Source: CAD feature listing. Evaluate the final solid. Frame: model axes, mm. A direction names the side the tool comes from. Round coordinates to 2 decimals unless told otherwise and drop trailing zeros. Loops run counter-clockwise (first coordinate to the right, second up) from the corner with the lowest first, then second, coordinate; pieces in that order, holes last. Notation, with made-up numbers: M -39,-32 L -11,-32 A17 ccw -11,-11 Z; hole C 45.5,-22.5 d1. An arc over 180 degrees is marked long. Answer as a JSON object with one key per item and string values.
from build123d import *

# Parameters (mm, degrees)
F1_DEPTH = 50.8
F3_DEPTH = 2.54
F4_W     = 170.18
F4_H     = 43.18
F5_DEPTH = 82.5510001


with BuildPart() as f1:
    # F0 (on Front) → F1 (new body)
    with BuildSketch(Plane.XZ):
        with BuildLine():
            Line((-89.1799991712, 82.55), (-89.1799991712, 0))
            Line((-89.1799991712, 0), (88.6200008288, 0))
            Line((88.6200008288, 0), (88.6200008288, 82.55))
            Line((88.6200008288, 82.55), (85.1941899427, 82.55))
            ThreePointArc((85.1941899427, 82.55), (0, 6.35), (-85.1941899427, 82.55))
            Line((-85.1941899427, 82.55), (-89.1799991712, 82.55))
        make_face()
    extrude(amount=F1_DEPTH)

    # F2 (on face) → F3 (cut)
    with BuildSketch(Plane.YZ.offset(88.6200008288)):
        Polygon((-37.5634527076, 56.1206514695), (-45.9675195587, 33.2813703549), (-43.8684808629, 33.2813703549), (-35.4644140118, 56.1206514695), align=None)
        Polygon((-37.9258376017, 33.2813703549), (-30.8785599801, 33.2813703549), (-22.4744931291, 56.1206514695), (-29.5217707507, 56.1206514695), align=None)
        Polygon((-34.8114763209, 56.1206514695), (-43.215543172, 33.2813703549), (-38.6183339685, 33.2813703549), (-30.2142671174, 56.1206514695), align=None)
        with BuildLine():
            Line((-21.8350046216, 56.1206514695), (-24.458008221, 48.992255464))
            Line((-24.458008221, 48.992255464), (-16.8186221192, 48.992255464))
            add(Edge.make_bspline(
                [(-16.8186221192, 48.992255464), (-16.5650688194, 48.7058519581), (-16.0364420635, 48.1087366521), (-16.1460089371, 46.764492626), (-16.7359200401, 45.358777375), (-17.0941465697, 45.0955807852), (-17.2307778252, 44.9951949189)],
                knots=[0, 0, 0, 0, 0.2524611124, 0.5263496824, 0.8193449335, 1, 1, 1, 1], degree=3))
            Line((-17.2307778252, 44.9951949189), (-25.8454084249, 44.9951949189))
            Line((-25.8454084249, 44.9951949189), (-28.7053373028, 37.2229198086))
            Line((-28.7053373028, 37.2229198086), (-22.3991661055, 25.6406514695))
            Line((-22.3991661055, 25.6406514695), (-12.5383959732, 25.6406514695))
            Line((-12.5383959732, 25.6406514695), (-10.2086553273, 33.3342202489))
            Line((-10.2086553273, 33.3342202489), (-15.8975594249, 33.3342202489))
            Line((-15.8975594249, 33.3342202489), (-18.6933472439, 38.4691212412))
            Line((-18.6933472439, 38.4691212412), (-12.1049555279, 38.4691212412))
            add(Edge.make_bspline(
                [(-10.4178804995, 56.1206514695), (-9.8079992001, 55.81468124), (-8.5579503395, 55.1875465219), (-7.2723425667, 53.2835881675), (-6.2681571478, 50.1731018561), (-6.5962499881, 46.920709582), (-7.4565458058, 43.3248722799), (-9.4576902901, 40.390709487), (-11.2329073266, 39.1021207418), (-12.1049555279, 38.4691212412)],
                knots=[0, 0, 0, 0, 0.1175129286, 0.2408614638, 0.3885970952, 0.5383784175, 0.6968239202, 0.8510693906, 1, 1, 1, 1], degree=3))
            Line((-10.4178804995, 56.1206514695), (-21.8350046216, 56.1206514695))
        make_face()
    extrude(amount=-F3_DEPTH, mode=Mode.SUBTRACT)

    # F4 (on face) → F5 (cut, through all)
    with BuildSketch(Plane(origin=(0, 0, 0), x_dir=(1, 0, 0), z_dir=(0, 0, -1))):
        with Locations((-0.2799991712, 25.4)):
            Rectangle(F4_W, F4_H)
    extrude(amount=-F5_DEPTH, mode=Mode.SUBTRACT)


solid = f1.part
Item 1: Pull-direction query (X, two-part tool) for faces 1 (the flat face through (86.08, -30, 45)), 2 (the flat face through (-7, -48, 0)), 3 (the flat face through (-89.18, -25, 42)), 4 (the flat face through (6, -3.81, 4)); classes: pulls with the +X half, pulls with the -X half, needs draft (parallel to the pull), parting line crosses it, or undercut.
Answer sheet:
{"face 1": "pulls with the +X half", "face 2": "needs draft", "face 3": "pulls with the -X half", "face 4": "undercut"}
Item 2: Section A-A on z = 65. Return the cut outline in (x, y), then the cut area to 3 significant figures.
Answer sheet:
{"outline": "M -89.18,-50.8 L -81.34,-50.8 L -81.34,-46.99 L -85.37,-46.99 L -85.37,-3.81 L -81.34,-3.81 L -81.34,0 L -89.18,0 Z; M 81.34,-50.8 L 88.62,-50.8 L 88.62,0 L 81.34,0 L 81.34,-3.81 L 84.81,-3.81 L 84.81,-46.99 L 81.34,-46.99 Z", "area": "444 mm²"}
Item 3: Section C-C on z = 16. Return the cut outline in (x, y).
Answer sheet:
{"outline": "M -89.18,-50.8 L -39.51,-50.8 L -39.51,-46.99 L -85.37,-46.99 L -85.37,-3.81 L -39.51,-3.81 L -39.51,0 L -89.18,0 Z; M 39.51,-50.8 L 88.62,-50.8 L 88.62,0 L 39.51,0 L 39.51,-3.81 L 84.81,-3.81 L 84.81,-46.99 L 39.51,-46.99 Z"}
Item 4: Section D-D on x = 76.5. Return the cut outline in (y, z), then the cut area to 3 significant figures.
Answer sheet:
{"outline": "M -50.8,0 L -46.99,0 L -46.99,53.39 L -50.8,53.39 Z; M -3.81,0 L 0,0 L 0,53.39 L -3.81,53.39 Z", "area": "407 mm²"}
Item 5: Access query for faces 5 (the flat face through (6, -46.99, 4)), 6 (the flat face through (87.368, -34.475, 44.541)), 7 (the cylindrical face through (0.58, -2.7, 6.35)). Directions: +Z, -Z, +X, -X, +Y, -Y. A direction counts if a zero-diameter tool reaches every point of the face in a straight line with its end or side. Return the directions, or none.
Answer sheet:
{"face 5": "+Z, -Z", "face 6": "+X", "face 7": "+Z, +Y, -Y"}
Item 6: Line query: probe 1 along X at (y, z) = (-32.5, 72); probe 2 along Y at (x, z) = (25, 7); probe 3 along X at (y, z) = (-29, 45). Output: solid intervals per line, ascending. Write a range as from..to.
Answer sheet:
{"probe 1": "x = -89.18..-85.37, 84.81..88.62", "probe 2": "y = -50.8..-46.99, -3.81..0", "probe 3": "x = -89.18..-85.37, 84.81..86.08"}
Item 7: Contact query for a flat-ended pin moving along its axis: pin 1 Ø0.8 at (x, y) = (86.5, -14) entering from -Z. Output: stop coordinate, or through.
Answer sheet:
{"pin 1": "stops at z = 0"}
Item 8: Section B-B on x = 53. Return the cut outline in (y, z).
Answer sheet:
{"outline": "M -50.8,0 L -46.99,0 L -46.99,24.7 L -50.8,24.7 Z; M -3.81,0 L 0,0 L 0,24.7 L -3.81,24.7 Z"}
